```python
from build123d import *

# Parameters (mm, degrees)
FILLET008_R               = 1
BOX003_W                  = 40
BOX003_H                  = 10
BOX003_DEPTH              = 10
FILLET007_R               = 1
BOX002_W                  = 39
BOX002_H                  = 15
BOX002_DEPTH              = 37
BOX001_W                  = 39
BOX001_H                  = 39
BOX001_DEPTH              = 15
BOX_W                     = 40
BOX_H                     = 40
BOX_DEPTH                 = 40
FILLET_R                  = 1
FILLET001_R               = 1
FILLET002_R               = 1
FILLET003_R               = 1
FILLET004_R               = 1
FILLET005_R               = 1
FILLET006_R               = 1
FILLET006_PLACEMENT_ANGLE = 180
FILLET009_R               = 1
FILLET010_R               = 1
FILLET011_R               = 1
FILLET012_R               = 1


with BuildPart() as fillet008:
    # Cone → Cone (revolve)
    with BuildSketch(Plane(origin=(35, -20, 15), x_dir=(1, 0, 0), z_dir=(0, -1, 0))):
        Polygon((0, 0), (5, 0), (2, 5), (0, 5), align=None)
    revolve(axis=Axis((35, -20, 15), (0, 0, 1)))

    # Fillet008
    fillet008_edges = [fillet008.edges().sort_by_distance(p)[0] for p in [
        (33, -20, 20),
    ]]
    fillet(fillet008_edges, radius=FILLET008_R)


with BuildPart() as fillet008_1:
    # Fillet008 placement: moved
    add(fillet008.part.moved(Location((-1, 0, 0))))


with BuildPart() as fillet007:
    # Box003 → Box003 (new body)
    with BuildSketch(Plane(origin=(0, -25, 5), x_dir=(1, 0, 0), z_dir=(0, 0, 1))):
        with Locations((20, 5)):
            Rectangle(BOX003_W, BOX003_H)
    extrude(amount=BOX003_DEPTH)

    # Fillet007
    fillet007_edges = [fillet007.edges().sort_by_distance(p)[0] for p in [
        (40, -25, 10),
        (40, -20, 15),
        (40, -15, 10),
        (40, -20, 5),
    ]]
    fillet(fillet007_edges, radius=FILLET007_R)


with BuildPart() as cube002:
    # Box002 → Box002 (new body)
    with BuildSketch(Plane(origin=(3, 3, 0), x_dir=(1, 0, 0), z_dir=(0, 0, 1))):
        with Locations((19.5, 7.5)):
            Rectangle(BOX002_W, BOX002_H)
    extrude(amount=BOX002_DEPTH)


with BuildPart() as cube001:
    # Box001 → Box001 (new body)
    with BuildSketch(Plane(origin=(3, 2, 22), x_dir=(1, 0, 0), z_dir=(0, 0, 1))):
        with Locations((19.5, 19.5)):
            Rectangle(BOX001_W, BOX001_H)
    extrude(amount=BOX001_DEPTH)


with BuildPart() as fusion001:
    # Box → Box (new body)
    with BuildSketch(Plane.XY):
        with Locations((20, 20)):
            Rectangle(BOX_W, BOX_H)
    extrude(amount=BOX_DEPTH)

    # Cut: cut Cube001
    add(cube001.part, mode=Mode.SUBTRACT)

    # Cut001: cut Cube002
    add(cube002.part, mode=Mode.SUBTRACT)

    # Fillet
    fillet_edges = [fusion001.edges().sort_by_distance(p)[0] for p in [
        (21.5, 18, 22),
    ]]
    fillet(fillet_edges, radius=FILLET_R)

    # Fillet001
    fillet001_edges = [fusion001.edges().sort_by_distance(p)[0] for p in [
        (21.5, 18, 0),
    ]]
    fillet(fillet001_edges, radius=FILLET001_R)

    # Fillet002
    fillet002_edges = [fusion001.edges().sort_by_distance(p)[0] for p in [
        (20, 40, 0),
        (21.5, 40, 22),
    ]]
    fillet(fillet002_edges, radius=FILLET002_R)

    # Fillet003
    fillet003_edges = [fusion001.edges().sort_by_distance(p)[0] for p in [
        (20, 0, 0),
        (0, 40, 20.5),
        (20, 40, 40),
        (0, 20, 40),
        (0, 0, 20),
        (40, 0, 20),
        (20, 0, 40),
        (40, 20, 40),
    ]]
    fillet(fillet003_edges, radius=FILLET003_R)

    # Fillet004
    fillet004_edges = [fusion001.edges().sort_by_distance(p)[0] for p in [
        (40, 3, 11),
    ]]
    fillet(fillet004_edges, radius=FILLET004_R)

    # Fillet005
    fillet005_edges = [fusion001.edges().sort_by_distance(p)[0] for p in [
        (40, 21, 37),
    ]]
    fillet(fillet005_edges, radius=FILLET005_R)

    # Fillet006
    fillet006_edges = [fusion001.edges().sort_by_distance(p)[0] for p in [
        (40, 40, 11),
        (40, 29, 0),
        (40, 29, 22),
        (40, 18, 11),
    ]]
    fillet(fillet006_edges, radius=FILLET006_R)


with BuildPart() as fusion001_1:
    # Fillet006 placement: moved
    add(fusion001.part.rotate(Axis((0, 0, 0), (0, 0, 1)), FILLET006_PLACEMENT_ANGLE))

    # Fusion: union Fillet007
    add(fillet007.part)

    # Fillet009
    fillet009_edges = [fusion001_1.edges().sort_by_distance(p)[0] for p in [
        (0, -20, 15),
    ]]
    fillet(fillet009_edges, radius=FILLET009_R)

    # Fillet010
    fillet010_edges = [fusion001_1.edges().sort_by_distance(p)[0] for p in [
        (0, -15, 10),
    ]]
    fillet(fillet010_edges, radius=FILLET010_R)

    # Fillet011
    fillet011_edges = [fusion001_1.edges().sort_by_distance(p)[0] for p in [
        (0, -25, 10),
    ]]
    fillet(fillet011_edges, radius=FILLET011_R)

    # Fillet012
    fillet012_edges = [fusion001_1.edges().sort_by_distance(p)[0] for p in [
        (0, -20, 5),
    ]]
    fillet(fillet012_edges, radius=FILLET012_R)

    # Fusion001: union Fillet008
    add(fillet008_1.part)


solid = fusion001_1.part
```
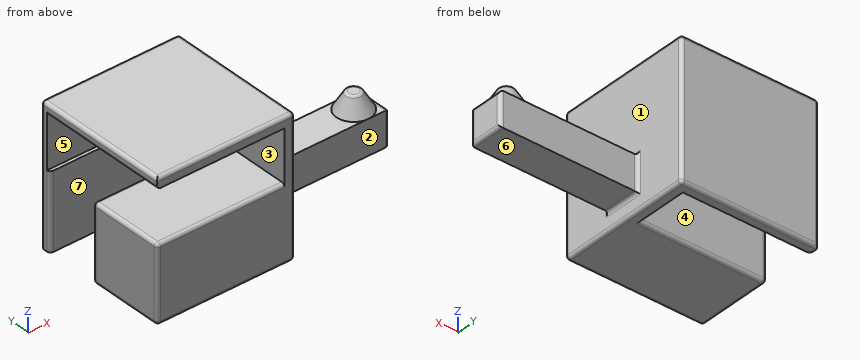
Design review of the part built by this model. Coordinates are the model's own, in mm. Face numbers are marked on the shaded views. A direction names the side the tool comes from. Coordinates: 2 decimals unless noted, no trailing zeros. Write each loop counter-clockwise with the first axis right and the second up, starting at its lowest first coordinate (ties: lowest second). Pieces come first, ordered by that corner, then holes.
1) Add section A-A (x = -27.5). Write out the cut boundary in (y, z), plus the area to 3 significant figures.
2) Add section B-B (y = -4). Write out the cut boundary in (x, z).
3) Insertion check: pin 1 (5.5 mm diameter, centred on x = 35.5, y = -22.5, fed in from +Z); pin 2 (11 mm diameter, centred on x = 29.5, z = 12, fed in from -Y); pin 3 (2 mm diameter, centred on y = -33, z = 18.5, fed in from +X); pin 4 (5 mm diameter, centred on x = 16.5, y = -28.5, fed in from +Z). Each pin has a flat end and moves straight along its axis. Give the tip position at first contact, or say it passes through.
4) To check wall thickness, follow L1, parallel to Z at x = -30, y = -19; L2, parallel to Y at x = -10.5, z = 15; L3, parallel to Y at x = 8.5, z = 10. State the ranges of each line that lie inside material, in increasing order.
5) Machinability: for the marked faces 5, 6 and 7, which of the approach directions +Z, -Z, +X, -X, +Y, -Y give a long, thin tool a straight path to every point of the face, cutting with its end or side? Answer none if there is none.
6) Add section D-D (x = 11). Write out the cut boundary in (y, z).
7) Add section C-C (z = 34). Write out the cut boundary in (x, y), plus the area to 3 significant figures.
8) Mouldability with a two-part tool opening along Y and no side actions: class the marked faces 1, 2, 3 and 4 as +Y half, -Y half, draft (parallel to the pull), parting line (faces both ways), or undercut.
Check result:
1. outline: (-40, 1) arc R1 ccw to (-39, 0) - (-19, 0) arc R1 ccw to (-18, 1) - (-18, 21) arc R1 ccw to (-19, 22) - (-39, 22) arc R1 ccw to (-40, 21) - close; (-40, 37) - (-2, 37) - (-2, 22) - (-3, 22) - (-3, 0) - (-1, 0) arc R1 ccw to (0, 1) - (0, 39) arc R1 ccw to (-1, 40) - (-39, 40) arc R1 ccw to (-40, 39) - close
1. area: 698 mm2
2. outline: (-40, 38) arc R1 ccw to (-39, 37) - (-3, 37) - (-3, 0) - (-1, 0) arc R1 ccw to (0, 1) - (0, 39) arc R1 ccw to (-1, 40) - (-39, 40) arc R1 ccw to (-40, 39) - close
3. pin 1: stops at z = 20
3. pin 2: stops at y = -25
3. pin 3: stops at x = 0
3. pin 4: passes through
4. L1: z = 0 to 22, 37 to 40
4. L2: y = -40 to -18, -3 to 0
4. L3: y = -25 to -15
5. face 5: -X, -Y
5. face 6: -Z, +X, +Y, -Y
5. face 7: -Z, -X
6. outline: (-25, 5) - (-15, 5) - (-15, 15) - (-25, 15) - close
7. outline: (-40, -2) - (-3, -2) - (-3, -40) - (-1, -40) arc R1 ccw to (0, -39) - (0, -1) arc R1 ccw to (-1, 0) - (-39, 0) arc R1 ccw to (-40, -1) - close
7. area: 193 mm2
8. face 1: draft
8. face 2: -Y half
8. face 3: undercut
8. face 4: undercut
